Geometry: final body of the model. Coordinates: model frame, mm. A direction names the side the tool comes from. Give positions to 0.01 mm unless a question says otherwise; leave off trailing zeros. Write each loop counter-clockwise with the first axis right and the second up, starting at its lowest first coordinate (ties: lowest second). Pieces come first, ordered by that corner, then holes. Notation, with made-up numbers: (-32, 44) -> (19, 44) arc R13 ccw to (19, 69) -> close; hole circle Ø8 at (81, -34). An arc over 180 degrees is marked (long way). Answer as a JSON object with one key per item and string values.
from build123d import *

# Parameters (mm, degrees)
F1_DEPTH = 41.275
F2_R     = 9.525
F3_DEPTH = 53.34
F5_DEPTH = 41.656
F7_DEPTH = 42.164
F8_R     = 1.5875
F9_DEPTH = 41.656


with BuildPart() as f1:
    # F0 (on Front) → F1 (new body)
    with BuildSketch(Plane.XZ):
        Polygon((304.8, 0), (304.8, 19.05), (0, 73.025), (0, 0), align=None)
    extrude(amount=-F1_DEPTH)

    # F2 (on face) → F3 (cut)
    with BuildSketch(Plane(origin=(0, 0, 0), x_dir=(0, -1, 0), z_dir=(-1, 0, 0))):
        with Locations((-20.6375, 36.5125)):
            Circle(F2_R)
    extrude(amount=-F3_DEPTH, mode=Mode.SUBTRACT)

    # F4 (on face) → F5 (cut)
    with BuildSketch(Plane.XZ):
        with BuildLine():
            ThreePointArc((0, 58.4309995174), (103.3439877315, 50.1875204766), (206.112158097, 36.5259720036))
            Line((206.112158097, 36.5259720036), (0, 73.025))
            Line((0, 73.025), (0, 58.4309995174))
        make_face()
        with BuildLine():
            Line((304.8, 19.05), (271.8913928646, 24.8775658469))
            ThreePointArc((271.8913928646, 24.8775658469), (291.3064644297, 16.355353839), (304.8, 0))
            Line((304.8, 0), (304.8, 19.05))
        make_face()
    extrude(amount=-F5_DEPTH, mode=Mode.SUBTRACT)

    # F6 (on face) → F7 (cut)
    with BuildSketch(Plane.XZ):
        with BuildLine():
            ThreePointArc((0, 53.1503558159), (29.1755322562, 54.9802482596), (58.4034793796, 54.4442484998))
            ThreePointArc((58.4034793796, 54.4442484998), (29.216529401, 56.6542842892), (0, 58.4309995174))
            Line((0, 58.4309995174), (0, 53.1503558159))
        make_face()
        with BuildLine():
            ThreePointArc((177.9886173747, 40.8118412298), (128.9105515624, 47.3016400104), (79.6850837991, 52.5578131014))
            ThreePointArc((79.6850837991, 52.5578131014), (128.2234853746, 41.5514956376), (177.9886173747, 40.8118412298))
        make_face()
    extrude(amount=-F7_DEPTH, mode=Mode.SUBTRACT)

    # F8 (on face) → F9 (cut)
    with BuildSketch(Plane.XZ):
        with Locations((30.00802733, 12.426703237)):
            Circle(F8_R)
        with Locations((267.163425684, 12.426703237)):
            Circle(F8_R)
    extrude(amount=-F9_DEPTH, mode=Mode.SUBTRACT)


solid = f1.part
Q1. First-contact query: P1, Ø12, axis at x = 221, z = 40.5, coming from the -Y side; P2, Ø11.5, axis at y = 20.64, z = 36.51, coming from the -X side. Flat tips, straight axial feed; report the tip coordinate or a pass-through.
Values:
{"P1": "through", "P2": "x = 53.34"}
Q2. Material intervals for L1, parallel to Z at x = 16, y = 9.5; L2, parallel to Z at x = 176.5, y = 30; L3, parallel to X at y = 20, z = 16, sorted ascending. Write a range as from..to.
Values:
{"L1": "0..54.45", "L2": "0..40.68", "L3": "0..291.77"}
Q3. Cut plane A-A (y = 38). Return the cut outline in (x, z) (1 decimal).
Values:
{"outline": "(0, 0) -> (304.8, 0) arc R45.8 ccw to (271.9, 24.9) -> (206.1, 36.5) arc R1972.6 ccw to (178, 40.8) arc R239.6 cw to (79.7, 52.6) arc R1972.6 ccw to (58.4, 54.4) arc R361.1 ccw to (0, 53.2) -> close; hole circle Ø3.2 at (30, 12.4); hole circle Ø3.2 at (267.2, 12.4)"}
Q4. Set-up query: faces 1 (the cylindrical face through (68.898, 20.349, 53.543)), 2 (the flat face through (53.34, 21, 37)). Return all of +Z, -Z, +X, -X, +Y, -Y with unobstructed straight access to the full face (end or side cutting, diameter ignored); none if empty.
Values:
{"face 1": "+Z, +X, +Y, -Y", "face 2": "-X"}
Q5. Cut plane C-C (y = 27). Return the cut outline in (x, z) (1 decimal).
Values:
{"outline": "(0, 0) -> (304.8, 0) arc R45.8 ccw to (271.9, 24.9) -> (206.1, 36.5) arc R1972.6 ccw to (178, 40.8) arc R239.6 cw to (79.7, 52.6) arc R1972.6 ccw to (58.4, 54.4) arc R361.1 ccw to (0, 53.2) -> (0, 43.6) -> (53.3, 43.6) -> (53.3, 29.4) -> (0, 29.4) -> close; hole circle Ø3.2 at (30, 12.4); hole circle Ø3.2 at (267.2, 12.4)"}
Q6. Mould query, pull axis Y, two halves, no side actions, for faces 3 (the flat face through (116, 41.275, 22)), 4 (the cylindrical face through (28.77, 20.35, 54.97)), 5 (the cylindrical face through (26.297, 15.517, 44.544)). Classes: pulls with the +Y half, pulls with the -Y half, needs draft (parallel to the pull), parting line crosses it, or undercut.
Values:
{"face 3": "pulls with the +Y half", "face 4": "needs draft", "face 5": "undercut"}
Q7. Cut plane D-D (z = 49). Return the cut outline in (x, y) (3 decimals), and give its area (3 significant figures).
Values:
{"outline": "(0, 0) -> (91.102, 0) -> (91.102, 41.275) -> (0, 41.275) -> close", "area": "3,760 mm²"}
